Autodesk Inventor part; units mm, degrees
ref_plane "YZ Plane" through (0, 0, 0) normal (1, 0, 0) x (0, 1, 0)
ref_plane "XZ Plane" through (0, 0, 0) normal (0, 1, 0) x (-1, 0, 0)
ref_plane "XY Plane" through (0, 0, 0) normal (0, 0, 1) x (1, 0, 0)
ref_plane "Work Plane2" through (35.545, -31.609, 1.6) normal (0, 0, 1) x (1, 0, 0)
sketch "Sketch2" plane through (35.545, -31.609, 1.6) normal (0, 0, 1) x (1, 0, 0)
  line L0 (-4.7778, 3.1171) -> (341.5466, 3.1925) construction
  line L1 (341.5466, 3.1925) -> (341.5765, -133.848) construction
  line L2 (341.5765, -133.848) -> (-4.7479, -133.9235) construction
  line L3 (-4.7479, -133.9235) -> (-4.7778, 3.1171) construction
  point P0 (-35.545, 31.609)
ref_plane "Work Plane1" through (371.545, -162.609, 0) normal (0, 0, -1) x (-1, 0, 0)
sketch "Sketch9" plane through (371.545, -162.609, 0) normal (0, 0, -1) x (-1, 0, 0)
  line L0 (336, 131) -> (0, 131)
  line L1 (-2, 129) -> (-2, 2)
  line L2 (-1.9796, 129.2846) -> (-2, 129)
  line L3 (-1.919, 129.5635) -> (-1.9796, 129.2846)
  line L4 (-1.8193, 129.8308) -> (-1.919, 129.5635)
  line L5 (-1.6825, 130.0813) -> (-1.8193, 129.8308)
  line L6 (-1.5115, 130.3097) -> (-1.6825, 130.0813)
  line L7 (-1.3097, 130.5115) -> (-1.5115, 130.3097)
  line L8 (-1.0813, 130.6825) -> (-1.3097, 130.5115)
  line L9 (-0.8308, 130.8193) -> (-1.0813, 130.6825)
  line L10 (-0.5635, 130.919) -> (-0.8308, 130.8193)
  line L11 (-0.2846, 130.9796) -> (-0.5635, 130.919)
  line L12 (0, 131) -> (-0.2846, 130.9796)
  circle A0 centre (2.362, 128.645) radius 1.1
  circle A1 centre (68.695, 128.645) radius 1.1
  circle A2 centre (135.028, 128.645) radius 1.1
  circle A3 centre (201.361, 128.645) radius 1.1
  circle A4 centre (267.694, 128.645) radius 1.1
  circle A5 centre (334.027, 128.645) radius 1.1
  line L13 (338, 2) -> (338, 129)
  line L14 (338, 129) -> (337.9796, 129.2846)
  line L15 (337.9796, 129.2846) -> (337.919, 129.5635)
  line L16 (337.919, 129.5635) -> (337.8193, 129.8308)
  line L17 (337.8193, 129.8308) -> (337.6825, 130.0813)
  line L18 (337.6825, 130.0813) -> (337.5115, 130.3097)
  line L19 (337.5115, 130.3097) -> (337.3097, 130.5115)
  line L20 (337.3097, 130.5115) -> (337.0813, 130.6825)
  line L21 (337.0813, 130.6825) -> (336.8308, 130.8193)
  line L22 (336.8308, 130.8193) -> (336.5635, 130.919)
  line L23 (336.5635, 130.919) -> (336.2846, 130.9796)
  line L24 (336.2846, 130.9796) -> (336, 131)
  line L25 (0, 0) -> (336, 0)
  line L26 (336, 0) -> (336.2846, 0.0204)
  line L27 (336.2846, 0.0204) -> (336.5635, 0.081)
  line L28 (336.5635, 0.081) -> (336.8308, 0.1807)
  line L29 (336.8308, 0.1807) -> (337.0813, 0.3175)
  line L30 (337.0813, 0.3175) -> (337.3097, 0.4885)
  line L31 (337.3097, 0.4885) -> (337.5115, 0.6903)
  line L32 (337.5115, 0.6903) -> (337.6825, 0.9187)
  line L33 (337.6825, 0.9187) -> (337.8193, 1.1692)
  line L34 (337.8193, 1.1692) -> (337.919, 1.4365)
  line L35 (337.919, 1.4365) -> (337.9796, 1.7154)
  line L36 (337.9796, 1.7154) -> (338, 2)
  circle A6 centre (334.02, 2.37) radius 1.1
  circle A7 centre (267.687, 2.37) radius 1.1
  circle A8 centre (201.354, 2.37) radius 1.1
  circle A9 centre (135.021, 2.37) radius 1.1
  circle A10 centre (68.688, 2.37) radius 1.1
  circle A11 centre (2.355, 2.37) radius 1.1
  line L37 (-0.2846, 0.0204) -> (0, 0)
  line L38 (-0.5635, 0.081) -> (-0.2846, 0.0204)
  line L39 (-0.8308, 0.1807) -> (-0.5635, 0.081)
  line L40 (-1.0813, 0.3175) -> (-0.8308, 0.1807)
  line L41 (-1.3097, 0.4885) -> (-1.0813, 0.3175)
  line L42 (-1.5115, 0.6903) -> (-1.3097, 0.4885)
  line L43 (-1.6825, 0.9187) -> (-1.5115, 0.6903)
  line L44 (-1.8193, 1.1692) -> (-1.6825, 0.9187)
  line L45 (-1.919, 1.4365) -> (-1.8193, 1.1692)
  line L46 (-1.9796, 1.7154) -> (-1.919, 1.4365)
  line L47 (-2, 2) -> (-1.9796, 1.7154)
  circle A12 centre (41.979, 103.44) radius 1.1
  circle A13 centre (125.979, 103.44) radius 1.1
  circle A14 centre (210.039, 103.527) radius 1.1
  circle A15 centre (294.039, 103.527) radius 1.1
  point P0 (371.545, 162.609)
ref_plane "Work Plane3" through (371.545, -162.609, 0) normal (0, 0, 1) x (1, 0, 0)
sketch "Sketch10" plane through (371.545, -162.609, 0) normal (0, 0, 1) x (1, 0, 0)
  circle A0 centre (-294.039, 103.527) radius 1.1
  circle A1 centre (-210.039, 103.527) radius 1.1
  circle A2 centre (-125.979, 103.44) radius 1.1
  circle A3 centre (-41.979, 103.44) radius 1.1
  line L0 (-294.039, 117.527) -> (-41.979, 117.527)
  line L1 (-27.979, 103.527) -> (-27.979, 103.527)
  line L2 (-41.979, 89.527) -> (-294.039, 89.527)
  line L3 (-308.039, 103.527) -> (-308.039, 103.527)
  arc A4 (-27.979, 103.527) -> (-41.979, 117.527) centre (-41.979, 103.527) ccw
  arc A5 (-41.979, 89.527) -> (-27.979, 103.527) centre (-41.979, 103.527) ccw
  arc A6 (-294.039, 117.527) -> (-308.039, 103.527) centre (-294.039, 103.527) ccw
  arc A7 (-308.039, 103.527) -> (-294.039, 89.527) centre (-294.039, 103.527) ccw
  point P0 (-371.545, 162.609)
  point P1 (-27.979, 103.527)
  dimension "d89" = 14
  dimension "d90" = 14
  dimension "d91" = 14
  dimension "d92" = 14
  dimension "d93" = 14
extrude "Extrusion4" add sketch "Sketch10" along normal blind 3
properties part number "foot2"
The listing builds one solid part. Answer for the finished solid, in the listing's coordinates (mm). Give positions to 0.01 mm unless a question says otherwise; leave off trailing zeros. Order: outer loops, then holes, each group sorted by start corner. A loop starts at its lowest first (then second) coordinate and runs counter-clockwise, first axis right, second up. Notation, with made-up numbers: (14, 56) -> (40, 56) arc R16 ccw to (40, 70) -> close; hole circle Ø5 at (83, 10.5). An arc over 180 degrees is marked (long way). Put each result on its own line as item: value.
Item 1: A cutting plane is placed at A-A on z = 2. Give the vertices of the cut face in (x, y).
Established:
outline: (77.51, -73.08) -> (329.57, -73.08) arc R14 ccw to (329.57, -45.08) -> (77.51, -45.08) arc R14 ccw to start; hole circle Ø2.2 at (77.51, -59.08); hole circle Ø2.2 at (161.51, -59.08); hole circle Ø2.2 at (245.57, -59.17); hole circle Ø2.2 at (329.57, -59.17)
Item 2: Straight lines are drawn through the part: line 1 (X direction, y = -60, z = 1.2); line 2 (X direction, y = -61, z = 0.5); line 3 (X direction, y = -47.75, z = 1). For each, find the intervals that lie inside material, in ascending order.
Established:
line 1: x = 63.54 to 76.9, 78.11 to 160.9, 162.11 to 244.85, 246.29 to 328.85, 330.29 to 343.54
line 2: x = 63.64 to 343.43
line 3: x = 69.28 to 337.79
Item 3: A cutting plane is placed at B-B on y = -67.5. Give the vertices of the cut face in (x, z).
Established:
outline: (66.32, 0) -> (340.75, 0) -> (340.75, 3) -> (66.32, 3) -> close
Item 4: A cutting plane is placed at C-C on y = -48. Give the vertices of the cut face in (x, z).
Established:
outline: (68.95, 0) -> (338.12, 0) -> (338.12, 3) -> (68.95, 3) -> close
